Autodesk Inventor part; units mm, degrees
ref_plane "YZ Plane" through (0, 0, 0) normal (1, 0, 0) x (0, 1, 0)
ref_plane "XZ Plane" through (0, 0, 0) normal (0, 1, 0) x (-1, 0, 0)
ref_plane "XY Plane" through (0, 0, 0) normal (0, 0, 1) x (1, 0, 0)
sketch "Boceto1" plane through (0, 0, 0) normal (0, 0, 1) x (1, 0, 0)
  line L0 (0, 0) -> (90, 0)
  line L1 (90, 0) -> (90, 180)
  line L2 (90, 180) -> (0, 180)
  line L3 (0, 180) -> (0, 0)
  line L4 (27.082, 144.48) -> (62.918, 144.48)
  line L5 (62.918, 144.48) -> (62.918, 122.39)
  line L6 (62.918, 122.39) -> (27.082, 122.39)
  line L7 (27.082, 122.39) -> (27.082, 144.48)
  point P0 (45, 144.48)
  dimension "d0" = 180
  dimension "d1" = 90
  dimension "d2" = 35.52
  dimension "d3" = 22.09
  dimension "d4" = 35.836
  dimension "d5" = 45
sketch "Boceto2" plane through (0, 0, 0) normal (0, 0, 1) x (1, 0, 0)
  line L0 (0, 0) -> (90, 0)
  line L1 (90, 0) -> (90, 180)
  line L2 (90, 180) -> (0, 180)
  line L3 (0, 180) -> (0, 0)
  dimension "d6" = 90
  dimension "d7" = 180
extrude "Extrusión1" add sketch "Boceto2" along normal blind 30
extrude "Extrusión2" add sketch "Boceto1" against normal blind 10 contours L4 L5 L6 L7
properties part number "MoldeDerechoPiezaInferiorBarco"
CAD build for the part. Positions are in the model's coordinates, mm. A direction names the side the tool comes from. Round coordinates to 2 decimals unless told otherwise and drop trailing zeros. Loops run counter-clockwise (first coordinate to the right, second up) from the corner with the lowest first, then second, coordinate; pieces in that order, holes last.
(1) Cut at D-D (y = 43.5). Give the cut face in (x, z), plus the area to 3 significant figures.
(2) Cut at A-A (y = 140.5). Give the cut face in (x, z).
(3) Which spindle directions (+Z, -Z, +X, -X, +Y, -Y) get a long thin tool onto all of the face, cutting with end or side? Do faces 1 (the flat face through (45, 144.48, -5)), 2 (the flat face through (45, 122.39, -5)), 3 (the flat face through (27.082, 133, -5)). Say none if no direction does.
(4) Wall check: line 1 along Z through (x, y) = (22, 53); line 2 along Y through (x, z) = (31, -6). Give the ranges that are in metal, low to high.
(5) Cut at B-B (x = 37.5). Give the cut face in (y, z), plus the area to 3 significant figures.
(6) Cut at C-C (x = 77). Give the cut face in (y, z), plus the area to 3 significant figures.
(7) Drop flat-ended pins along their axis: pin 1 (11 mm diameter, centred on y = 131, z = -4.5, fed in from -X); pin 2 (4 mm diameter, centred on x = 74.5, y = 26.5, fed in from -Z); pin 3 (8 mm diameter, centred on x = 50, z = -4.5, fed in from -Y); pin 4 (8 mm diameter, centred on x = 42.5, z = -6.5, fed in from +Y). Give the stop position or say it passes through.
Findings below:
1. outline: (0, 0) - (90, 0) - (90, 30) - (0, 30) - close
1. area: 2,700 mm2
2. outline: (0, 0) - (27.08, 0) - (27.08, -10) - (62.92, -10) - (62.92, 0) - (90, 0) - (90, 30) - (0, 30) - close
3. face 1: -Z, +X, -X, +Y
3. face 2: -Z, +X, -X, -Y
3. face 3: -Z, -X, +Y, -Y
4. line 1: z = 0 to 30
4. line 2: y = 122.39 to 144.48
5. outline: (0, 0) - (122.39, 0) - (122.39, -10) - (144.48, -10) - (144.48, 0) - (180, 0) - (180, 30) - (0, 30) - close
5. area: 5,620 mm2
6. outline: (0, 0) - (180, 0) - (180, 30) - (0, 30) - close
6. area: 5,400 mm2
7. pin 1: stops at x = 0
7. pin 2: stops at z = 0
7. pin 3: stops at y = 122.39
7. pin 4: stops at y = 144.48
